```python
from build123d import *

# Parameters (mm, degrees)
SKETCH1_R           = 47.5
BOSS_EXTRUDE1_DEPTH = 20
FILLET1_R           = 45


with BuildPart() as part:
    # Sketch1 → Boss-Extrude1 (new body)
    with BuildSketch(Plane.XY):
        Polygon((-194.485228659, -273.050238686), (93.403745832, -273.050238686), (93.403745832, -345.680466299), (149.459258586, -304.039615326), (149.459258586, -273.050238686), (149.459258586, 26.949761314), (-50.540741414, 389.92600238), (-250.540741414, 26.949761314), (-250.540741414, -273.050238686), (-250.540741414, -304.039615326), (-194.485228659, -345.680466299), align=None)
        with Locations((-50.540741414, -66.594312027)):
            Circle(SKETCH1_R, mode=Mode.SUBTRACT)
        Polygon((-220.540741414, -174.094312027), (-177.031307775, -174.094312027), (-220.540741414, -232.665247906), align=None, mode=Mode.SUBTRACT)
        Polygon((-88.038179167, -254.669001578), (-147.89310645, -174.094312027), (46.811623623, -174.094312027), (-13.043303661, -254.669001578), align=None, mode=Mode.SUBTRACT)
        Polygon((89.802053233, -243.050238686), (32.959395338, -243.050238686), (61.380724285, -204.790401769), align=None, mode=Mode.SUBTRACT)
        Polygon((-220.540741414, -144.094312027), (-177.031307775, -144.094312027), (-177.031307775, -94.25920837), (-177.031307775, -51.592409031), (-177.031307775, 10.905687973), (-220.540741414, 10.905687973), (-220.540741414, -51.592409031), (-220.540741414, -94.25920837), align=None, mode=Mode.SUBTRACT)
        Polygon((-64.881138394, 251.355896711), (-116.293954083, 174.236673178), (-64.881138394, 174.236673178), align=None, mode=Mode.SUBTRACT)
        Polygon((93.403745832, 56.949761314), (33.381498462, 146.983132367), (-20.768536019, 56.949761314), align=None, mode=Mode.SUBTRACT)
        Polygon((-194.485228659, 56.949761314), (-80.312946809, 56.949761314), (-134.46298129, 146.983132367), align=None, mode=Mode.SUBTRACT)
        Polygon((119.459258586, -232.665247906), (75.949824948, -174.094312027), (119.459258586, -174.094312027), align=None, mode=Mode.SUBTRACT)
        Polygon((119.459258586, -144.094312027), (119.459258586, -94.25920837), (119.459258586, -51.592409031), (119.459258586, 10.905687973), (75.949824948, 10.905687973), (75.949824948, -51.592409031), (75.949824948, -94.25920837), (75.949824948, -144.094312027), align=None, mode=Mode.SUBTRACT)
        Polygon((-190.883536061, -243.050238686), (-134.040878165, -243.050238686), (-162.462207113, -204.790401769), align=None, mode=Mode.SUBTRACT)
        with BuildLine():
            Line((-156.167658148, 10.905687973), (-156.167658148, -42.439597831))
            Line((-156.167658148, -42.439597831), (-124.18040316, -42.439597831))
            ThreePointArc((-124.18040316, -42.439597831), (-107.419195748, -13.953154816), (-80.312946809, 4.958925397))
            Line((-80.312946809, 4.958925397), (-80.312946809, 10.905687973))
            Line((-80.312946809, 10.905687973), (-156.167658148, 10.905687973))
        make_face(mode=Mode.SUBTRACT)
        with BuildLine():
            Line((-156.167658148, -144.094312027), (-156.167658148, -89.328160682))
            Line((-156.167658148, -89.328160682), (-124.631375946, -89.328160682))
            ThreePointArc((-124.631375946, -89.328160682), (-107.922842799, -118.686004653), (-80.312946809, -138.147549452))
            Line((-80.312946809, -138.147549452), (-80.312946809, -144.094312027))
            Line((-80.312946809, -144.094312027), (-156.167658148, -144.094312027))
        make_face(mode=Mode.SUBTRACT)
        with BuildLine():
            Line((-20.768536019, -138.147549452), (-20.768536019, -144.094312027))
            Line((-20.768536019, -144.094312027), (55.08617532, -144.094312027))
            Line((55.08617532, -144.094312027), (55.08617532, -89.328160682))
            Line((55.08617532, -89.328160682), (23.549893118, -89.328160682))
            ThreePointArc((23.549893118, -89.328160682), (6.841359971, -118.686004653), (-20.768536019, -138.147549452))
        make_face(mode=Mode.SUBTRACT)
        with BuildLine():
            Line((-20.768536019, 4.958925397), (-20.768536019, 10.905687973))
            Line((-20.768536019, 10.905687973), (55.08617532, 10.905687973))
            Line((55.08617532, 10.905687973), (55.08617532, -42.439597831))
            Line((55.08617532, -42.439597831), (23.098920333, -42.439597831))
            ThreePointArc((23.098920333, -42.439597831), (6.337712921, -13.953154816), (-20.768536019, 4.958925397))
        make_face(mode=Mode.SUBTRACT)
        Polygon((13.443150149, 158.032314781), (-36.200344433, 158.032314781), (-36.200344433, 75.49181022), align=None, mode=Mode.SUBTRACT)
        Polygon((15.212471256, 174.236673178), (-36.200344433, 251.355896711), (-36.200344433, 174.236673178), align=None, mode=Mode.SUBTRACT)
        Polygon((-114.524632976, 158.032314781), (-64.881138394, 75.49181022), (-64.881138394, 158.032314781), align=None, mode=Mode.SUBTRACT)
    extrude(amount=BOSS_EXTRUDE1_DEPTH)

    # Fillet1
    fillet1_edges = [part.edges().sort_by_distance(p)[0] for p in [
        (149.459258586, -304.039615326, 10),
        (-250.540741414, -304.039615326, 10),
        (-250.540741414, 26.949761314, 10),
        (-50.540741414, 389.92600238, 10),
        (149.459258586, 26.949761314, 10),
    ]]
    fillet(fillet1_edges, radius=FILLET1_R)


solid = part.part
```
Can you work these out from the model? Positions are in its coordinate system, mm. A direction names the side the tool comes from. Coordinates: 2 decimals unless noted, no trailing zeros. Loops run counter-clockwise (first coordinate to the right, second up) from the corner with the lowest first, then second, coordinate; pieces in that order, holes last. Notation, with made-up numbers: (71.25, 15) -> (87.25, 15) arc R14 ccw to (87.25, 42) -> close; hole circle Ø11 at (-3.75, 51.5). An arc over 180 degrees is marked (long way). Put each result on its own line as item: value. Start each with the question number.
Q1. For faces 4 (the face through (93.404, -309, 10)), 5 (the face through (148.08, 26.43, 10.14)), 6 (the face through (119.459, -66, 10)), which set-ups out of +Z, -Z, +X, -X, +Y, -Y let a thin tool reach every point of the face, with its end or its side?
Q2. I'm going to push flat-ended pins straight in: P1, Ø4, axis at x = -99.5, z = 6, coming from the +Y side; P2, Ø5, axis at y = 212.5, z = 16.5, coming from the +X side; P3, Ø1, axis at x = 15, z = 8, coming from the +Y side. Where does each tip first touch, or does it pass through?
Q3. If I drill on line 1 (X direction, y = -67.5, z = 5); line 2 (Y direction, x = -186, z = 13); line 3 (X direction, y = -17.5, z = 19), over which ranges is the centre line in solid material (lowest first)? Write a range as [from, to].
Q4. I want a section at D-D (z = 13). Count the separate pieces of the cut face and the enclosed holes in it, plus the area to 3 significant figures.
Q5. I want a section at B-B (x = 108.5). Write out the boundary of the cut face in (y, z).
Q6. I want a section at A-A (y = 99). Write out the boundary of the cut face in (x, z), plus the area to 3 significant figures.
Q7. I want a section at C-C (y = 193). Write out the boundary of the cut face in (x, z).
Q8. Thinking about a two-plate mould opening in Y: for faces 1 (the face through (-249.16, 26.43, 10.14)), 2 (the face through (6.686, 102.597, 9.86)), 3 (the face through (112.083, -331.804, 9.86)), which applies, pulls with the +Y half, pulls with the -Y half, needs draft (parallel to the pull), parting line crosses it, or undercut?
Taken from the geometry:
1. face 4: +Z, -Z, -Y
1. face 5: +Z, -Z, +X, +Y
1. face 6: +Z, -Z
2. P1: stops at y = 304.7
2. P2: stops at x = 48.6
2. P3: stops at y = 271.88
3. line 1: x = [-250.54, -220.54], [-177.03, -98.03], [-3.05, 75.95], [119.46, 149.46]
3. line 2: y = [-273.05, -243.05], [-236.48, -186.17], [-174.09, -144.09], [10.91, 56.95], [69.68, 144.08]
3. line 3: x = [-250.54, -220.54], [-177.03, -156.17], [-110.51, 9.43], [55.09, 75.95], [119.46, 149.46]
4. separate pieces: 1
4. enclosed holes: 18
4. area: 131,000 mm2
5. outline: (-334.47, 0) -> (-217.91, 0) -> (-217.91, 20) -> (-334.47, 20) -> close; (-174.09, 0) -> (-144.09, 0) -> (-144.09, 20) -> (-174.09, 20) -> close; (10.91, 0) -> (101.29, 0) -> (101.29, 20) -> (10.91, 20) -> close
6. outline: (-210.84, 0) -> (-166.45, 0) -> (-166.45, 20) -> (-210.84, 20) -> close; (-105.6, 0) -> (-79.02, 0) -> (-79.02, 20) -> (-105.6, 20) -> close; (-64.88, 0) -> (-36.2, 0) -> (-36.2, 20) -> (-64.88, 20) -> close; (-22.06, 0) -> (4.52, 0) -> (4.52, 20) -> (-22.06, 20) -> close; (65.37, 0) -> (109.76, 0) -> (109.76, 20) -> (65.37, 20) -> close
6. area: 3,410 mm2
7. outline: (-159.05, 0) -> (-103.79, 0) -> (-103.79, 20) -> (-159.05, 20) -> close; (-64.88, 0) -> (-36.2, 0) -> (-36.2, 20) -> (-64.88, 20) -> close; (2.7, 0) -> (57.97, 0) -> (57.97, 20) -> (2.7, 20) -> close
8. face 1: pulls with the +Y half
8. face 2: undercut
8. face 3: pulls with the -Y half
